Could you check a few things on this model? Use its own coordinates, in mm. A direction names the side the tool comes from. Give positions to 0.01 mm unless a question says otherwise; leave off trailing zeros. Loops run counter-clockwise (first coordinate to the right, second up) from the corner with the lowest first, then second, coordinate; pieces in that order, holes last. Notation, with made-up numbers: (-17, -10.5) -> (37, -10.5) arc R21 cw to (37, 13.5) -> close; hole circle Ø2 at (-16.75, 31). An arc over 180 degrees is marked (long way). Write item = value, one per line. Start each with the question number.
1) I need wall thicknesses on probe 1 along Y at (x, z) = (32, 2.1); probe 2 along Y at (x, z) = (20.5, 1.1); probe 3 along Z at (x, y) = (11.5, -9). Which ranges of each line are inside material? Lowest first, please. Write a range as from..to.
2) I want a section at C-C (y = -8). List the corners of the cut face in (x, z) for me.
3) I want a section at B-B (x = 5). List the corners of the cut face in (y, z) for me, and give its area (4 significant figures).
4) On a 3-axis mill with a long thin cutter (end or side, diameter ignored), from which of +Z, -Z, +X, -X, +Y, -Y can I reach the whole of each face in a straight line? I mean faces 5 (the face through (-9.85, -12.57, -1.48)), 6 (the face through (-48.5, -16.57, 1.73)). Say none if no direction works.
5) I'm going to push a flat-ended pin straight in: pin 1 Ø4 at (x, y) = (32, 16.5) entering from -Z. Where does the tip first touch, or does it pass through?
6) I want a section at A-A (z = -1.5). List the corners of the cut face in (x, y) for me.
7) If we mould it in two halves opening along X, with no side actions, what happens to faces 1 (the face through (-50.147, -19.717, 1.726)), 2 (the face through (-1.194, 1.735, 1.726)), 3 (the face through (35.217, -19.647, 1.726)), 4 (the face through (-8.2, -2.1, 1.7))? For each: +X half, -X half, draft (parallel to the pull), parting line (faces both ways), or undercut.
8) I want a section at D-D (x = -29). List the corners of the cut face in (y, z) for me, and give its area (3 significant figures).
Autodesk Inventor part; units mm, degrees
ref_plane "YZ Plane" through (0, 0, 0) normal (1, 0, 0) x (0, 1, 0)
ref_plane "XZ Plane" through (0, 0, 0) normal (0, 1, 0) x (-1, 0, 0)
ref_plane "XY Plane" through (0, 0, 0) normal (0, 0, 1) x (1, 0, 0)
sketch "Sketch1" plane through (0, 0, 0) normal (0, 0, 1) x (1, 0, 0)
  line L0 (21.5, 21) -> (-21.5, 21)
  arc A0 (-21.5, 21) -> (-26, 16.5) centre (-21.5, 16.5) ccw construction
  line L1 (-26, 16.5) -> (-26, -16.5) construction
  arc A1 (-26, -16.5) -> (-21.5, -21) centre (-21.5, -16.5) ccw construction
  line L2 (-21.5, -21) -> (21.5, -21)
  arc A2 (21.5, -21) -> (26, -16.5) centre (21.5, -16.5) ccw construction
  line L3 (26, -16.5) -> (26, 16.5) construction
  arc A3 (26, 16.5) -> (21.5, 21) centre (21.5, 16.5) ccw construction
  circle A4 centre (5, 0) radius 2.5
  circle A5 centre (-20, 15.5) radius 1.5
  circle A6 centre (-10.5, -15.5) radius 1.2295
  circle A7 centre (-10.5, 15.5) radius 1.2295
  circle A8 centre (-2, 3) radius 1.5
  circle A9 centre (-2, -3) radius 1.5
  circle A10 centre (-7, 3) radius 1.5
  circle A11 centre (-7, -3) radius 1.5
  circle A12 centre (-12, 3) radius 1.5
  circle A13 centre (-12, -3) radius 1.5
  circle A14 centre (-20, -15.5) radius 1.5
  circle A15 centre (20.5, -15.5) radius 1.2295
  circle A16 centre (20.5, 15.5) radius 1.2295
  line L4 (-21.5, 21) -> (-47, 21)
  line L5 (-51.5, 16.5) -> (-51.5, -16.5)
  line L6 (-47, -21) -> (-21.5, -21)
  arc A17 (-47, 21) -> (-51.5, 16.5) centre (-47, 16.5) ccw
  arc A18 (-51.5, -16.5) -> (-47, -21) centre (-47, -16.5) ccw
  circle A19 centre (-47, -16.5) radius 1.5
  circle A20 centre (-47, 16.5) radius 1.5
  line L7 (21.5, 21) -> (32, 21)
  line L8 (36.5, 16.5) -> (36.5, -16.5)
  line L9 (32, -21) -> (21.5, -21)
  arc A21 (36.5, 16.5) -> (32, 21) centre (32, 16.5) ccw
  arc A22 (32, -21) -> (36.5, -16.5) centre (32, -16.5) ccw
  circle A23 centre (32, 16.5) radius 1.5
  circle A24 centre (32, -16.5) radius 1.5
  point P0 (0, 0)
  point P1 (-51.5, 21)
  point P2 (36.5, 21)
  dimension "d0" = 30
  dimension "d1" = 4.5
  dimension "d2" = 3
  dimension "d3" = 3
  dimension "d13" = 15
  dimension "d14" = 4.5
  dimension "d15" = 3
  dimension "d16" = 3
extrude "Extrusion1" add sketch "Sketch1" along normal blind 3.5
ref_plane "Work Plane1" through (0, 0, 10.75) normal (0, 0, -1) x (-1, 0, 0)
sketch "Sketch2" plane through (0, 0, 0) normal (0, 0, -1) x (-1, 0, 0)
  circle A0 centre (-20.5, 15.5) radius 1.2295
  circle A1 centre (-20.5, 15.5) radius 3
  circle A2 centre (10.5, 15.5) radius 1.2295
  circle A3 centre (10.5, 15.5) radius 3
  circle A4 centre (-20.5, -15.5) radius 1.2295
  circle A5 centre (-20.5, -15.5) radius 3
  circle A6 centre (10.5, -15.5) radius 1.2295
  circle A7 centre (10.5, -15.5) radius 3
  point P0 (0, 0)
  dimension "d7" = 6
  dimension "d8" = 6
  dimension "d9" = 6
  dimension "d10" = 6
extrude "Extrusion2" add sketch "Sketch2" along normal blind 3
equation "\"d7\" = d8"
equation "\"d9\" = d8"
equation "\"d10\" = d8"
properties part number "housingBack" material "ABS Plastic"
Answer list:
q1.probe_1 = -21..-18, -15..15, 18..21
q1.probe_2 = -21..-16.73, -14.27..14.27, 16.73..21
q1.probe_3 = 0..3.5
q2.outline = (-51.5, 0) -> (36.5, 0) -> (36.5, 3.5) -> (-51.5, 3.5) -> close
q3.outline = (-21, 0) -> (-2.5, 0) -> (-2.5, 3.5) -> (-21, 3.5) -> close; (2.5, 0) -> (21, 0) -> (21, 3.5) -> (2.5, 3.5) -> close
q3.area = 129.5 mm^2
q4.face_5 = -Z
q4.face_6 = +Z, -Z
q5.pin_1 = 0
q6.outline = circle Ø6 at (-10.5, -15.5); circle Ø6 at (-10.5, 15.5); circle Ø6 at (20.5, -15.5); circle Ø6 at (20.5, 15.5); hole circle Ø2.46 at (-10.5, -15.5); hole circle Ø2.46 at (-10.5, 15.5); hole circle Ø2.46 at (20.5, -15.5); hole circle Ø2.46 at (20.5, 15.5)
q7.face_1 = -X half
q7.face_2 = undercut
q7.face_3 = +X half
q7.face_4 = undercut
q8.outline = (-21, 0) -> (21, 0) -> (21, 3.5) -> (-21, 3.5) -> close
q8.area = 147 mm^2
